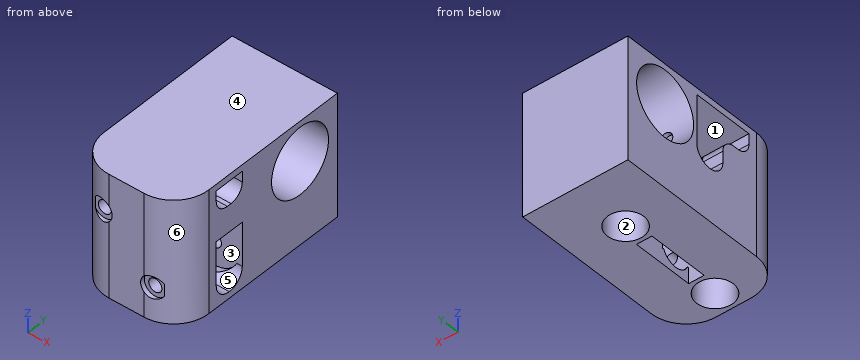
```python
from build123d import *

# Parameters (mm, degrees)
SKETCH_1_W           = 24
SKETCH_1_H           = 36
EXTRUDE_1_DEPTH      = 19
CUT_EXTRUDE_2_DEPTH  = 3.5
SKETCH_4_W           = 5.4
SKETCH_4_H           = 7
CUT_EXTRUDE_3_DEPTH  = 36.510561809
CUT_EXTRUDE_4_DEPTH  = 3.5
SKETCH_6_R           = 4.15
CUT_EXTRUDE_5_DEPTH  = 44.726422218
FILLET_2_R           = 3
SKETCH_10_W          = 10
SKETCH_10_H          = 36
CUT_EXTRUDE_9_DEPTH  = 36.510561809
SKETCH_11_W          = 28
SKETCH_11_H          = 16.5
EXTRUDE_3_DEPTH      = 24
SKETCH_12_W          = 10.25
SKETCH_12_H          = 12
EXTRUDE_4_DEPTH      = 7
FILLET_3_R           = 3.5
SKETCH_13_W          = 10.25
SKETCH_13_H          = 1.5
EXTRUDE_5_DEPTH      = 7
FILLET_4_R           = 3.5
SKETCH_14_R          = 5.6
CUT_EXTRUDE_10_DEPTH = 7
FILLET_6_R           = 3
EXTRUDE_START        = -18
SKETCH_16_R          = 4.15
EXTRUDE_6_DEPTH      = 18
SKETCH_17_R          = 7.65
SKETCH_17_W          = 28
SKETCH_17_H          = 17.5
SKETCH_17_H_2        = 9
CUT_EXTRUDE_11_DEPTH = 47.122120558
FILLET_7_R           = 8
SKETCH_18_R          = 1.5
CUT_EXTRUDE_12_DEPTH = 26
SKETCH_19_R          = 1.5
CUT_EXTRUDE_13_DEPTH = 20
SKETCH_20_R          = 2.5
CUT_EXTRUDE_14_DEPTH = 1


with BuildPart() as part:
    # 草图1 → 凸台-拉伸1 (new, symmetric)
    with BuildSketch(Plane.XY):
        Rectangle(SKETCH_1_W, SKETCH_1_H)
    extrude(amount=EXTRUDE_1_DEPTH, both=True)

    # 草图3 → 切除-拉伸2 (cut, symmetric)
    with BuildSketch(Plane(origin=(0, 3.5, 0), x_dir=(1, 0, 0), z_dir=(0, 1, 0))):
        with BuildLine():
            Line((-5.75, -7.5), (-12, -7.5))
            Line((-12, -7.5), (-12, 19))
            Line((-12, 19), (1.75, 19))
            Line((1.75, 19), (1.75, 0))
            ThreePointArc((1.75, 0), (-0.446699141, -5.303300859), (-5.75, -7.5))
        make_face()
    extrude(amount=CUT_EXTRUDE_2_DEPTH, both=True, mode=Mode.SUBTRACT)

    # 草图4 → 切除-拉伸3 (cut, through all)
    with BuildSketch(Plane.ZY.offset(12)):
        with Locations((4.8, -3.5)):
            Rectangle(SKETCH_4_W, SKETCH_4_H)
    extrude(amount=-CUT_EXTRUDE_3_DEPTH, mode=Mode.SUBTRACT)

    # 草图5 → 切除-拉伸4 (cut, symmetric)
    with BuildSketch(Plane(origin=(0, -3.5, 0), x_dir=(1, 0, 0), z_dir=(0, 1, 0))):
        with BuildLine():
            Line((5.75, 4), (12, 4))
            Line((12, 4), (12, 19))
            Line((12, 19), (-1.75, 19))
            Line((-1.75, 19), (-1.75, 11.5))
            ThreePointArc((-1.75, 11.5), (0.446699141, 6.196699141), (5.75, 4))
        make_face()
    extrude(amount=CUT_EXTRUDE_4_DEPTH, both=True, mode=Mode.SUBTRACT)

    # 草图6 → 切除-拉伸5 (cut, through all)
    with BuildSketch(Plane(origin=(0, 0, -19), x_dir=(-1, 0, 0), z_dir=(0, 0, -1))):
        with Locations((0, 12)):
            Circle(SKETCH_6_R)
        with Locations(Location((0, -12, 0), (0, 0, 180))):
            Circle(SKETCH_6_R)
    extrude(amount=-CUT_EXTRUDE_5_DEPTH, mode=Mode.SUBTRACT)

    # 圆角2
    fillet_2_edges = [part.edges().sort_by_distance(p)[0] for p in [
        (6.725, 0, 2.1),
        (0, -7, 2.1),
    ]]
    fillet(fillet_2_edges, radius=FILLET_2_R)

    # 草图10 → 切除-拉伸9 (cut, through all)
    with BuildSketch(Plane(origin=(12, 0, 0), x_dir=(0, 0, -1), z_dir=(1, 0, 0))):
        with Locations((-14, 0)):
            Rectangle(SKETCH_10_W, SKETCH_10_H)
    extrude(amount=-CUT_EXTRUDE_9_DEPTH, mode=Mode.SUBTRACT)

    # 草图11 → 凸台-拉伸3 (add)
    with BuildSketch(Plane.ZY.offset(12)):
        with Locations((-5, -26.25)):
            Rectangle(SKETCH_11_W, SKETCH_11_H)
    extrude_3 = extrude(amount=-EXTRUDE_3_DEPTH)

    # 镜向2: 凸台-拉伸3 across plane
    add(extrude_3.mirror(Plane.ZX))

    # 草图12 → 凸台-拉伸4 (add)
    with BuildSketch(Plane(origin=(0, 0, 0), x_dir=(1, 0, 0), z_dir=(0, 1, 0))):
        with Locations((-6.875, 13)):
            Rectangle(SKETCH_12_W, SKETCH_12_H)
    extrude(amount=EXTRUDE_4_DEPTH)

    # 圆角3
    fillet_3_edges = [part.edges().sort_by_distance(p)[0] for p in [
        (-6.875, 0, -7),
        (-6.875, 7, -7),
    ]]
    fillet(fillet_3_edges, radius=FILLET_3_R - 0.0001)  # a hair under: the kernel refuses the full size

    # 草图13 → 凸台-拉伸5 (add)
    with BuildSketch(Plane.XZ):
        with Locations((6.875, -18.25)):
            Rectangle(SKETCH_13_W, SKETCH_13_H)
    extrude(amount=EXTRUDE_5_DEPTH)

    # 圆角4
    fillet_4_edges = [part.edges().sort_by_distance(p)[0] for p in [
        (6.875, 0, -17.5),
        (6.875, -7, -17.5),
    ]]
    fillet(fillet_4_edges, radius=FILLET_4_R - 0.0001)  # a hair under: the kernel refuses the full size

    # 草图14 → 切除-拉伸10 (cut)
    with BuildSketch(Plane.XZ):
        with Locations((5.75, -11.5)):
            Circle(SKETCH_14_R)
    extrude(amount=CUT_EXTRUDE_10_DEPTH, mode=Mode.SUBTRACT)

    # 圆角6
    fillet_6_edges = [part.edges().sort_by_distance(p)[0] for p in [
        (-5.275, 0, 2.1),
    ]]
    fillet(fillet_6_edges, radius=FILLET_6_R)

    # 草图16 → 凸台-拉伸6 (add)
    with BuildSketch(Plane.XY.offset(9).offset(EXTRUDE_START)):
        with Locations((0, -12)):
            Circle(SKETCH_16_R)
        with Locations(Location((0, 12, 0), (0, 0, 180))):
            Circle(SKETCH_16_R)
    extrude(amount=EXTRUDE_6_DEPTH)

    # 草图17 → 切除-拉伸11 (cut, through all)
    with BuildSketch(Plane.ZY.offset(12)):
        with Locations(Location((0, 15.5, 0), (0, 0, 270))):
            Circle(SKETCH_17_R)
        with Locations((-5, -25.75)):
            Rectangle(SKETCH_17_W, SKETCH_17_H)
        with Locations((-5, 30)):
            Rectangle(SKETCH_17_W, SKETCH_17_H_2)
    extrude(amount=-CUT_EXTRUDE_11_DEPTH, mode=Mode.SUBTRACT)

    # 圆角7
    fillet_7_edges = [part.edges().sort_by_distance(p)[0] for p in [
        (12, -17, -5),
        (-12, -17, -5),
    ]]
    fillet(fillet_7_edges, radius=FILLET_7_R)

    # 草图18 → 切除-拉伸12 (cut)
    with BuildSketch(Plane.XZ.offset(17)):
        with Locations((-5.75, 0)):
            Circle(SKETCH_18_R)
    extrude(amount=-CUT_EXTRUDE_12_DEPTH, mode=Mode.SUBTRACT)

    # 草图19 → 切除-拉伸13 (cut)
    with BuildSketch(Plane.XZ.offset(17)):
        with Locations((5.75, -11.5)):
            Circle(SKETCH_19_R)
    extrude(amount=-CUT_EXTRUDE_13_DEPTH, mode=Mode.SUBTRACT)

    # 草图20 → 切除-拉伸14 (cut)
    with BuildSketch(Plane.XZ.offset(17)):
        with Locations((5.75, -11.5)):
            Circle(SKETCH_20_R)
        with Locations((-5.75, 0)):
            Circle(SKETCH_20_R)
    extrude(amount=-CUT_EXTRUDE_14_DEPTH, mode=Mode.SUBTRACT)


solid = part.part
```
Could you check a few things on this model? Use its own coordinates, in mm. Face numbers are marked on the shaded views. A direction names the side the tool comes from. Give positions to 0.01 mm unless a question says otherwise; leave off trailing zeros. Order: outer loops, then holes, each group sorted by start corner. A loop starts at its lowest first (then second) coordinate and runs counter-clockwise, first axis right, second up.
Q1. For the marked faces 1, 2 and 3, which set-ups out of +Z, -Z, +X, -X, +Y, -Y let a thin tool reach every point of the face, with its end or its side?
Q2. Suppose I cut it at D-D, the plane z = -8.5. Write out the boundary of the cut face in (x, y).
Q3. If I drill on line 1 along Y through (x, z) = (0, -11.75); line 2 along X through (y, z) = (12, -12.25); line 3 along Y through (x, z) = (2, -0.25), over which ranges is the centre line in solid material (lowest first)?
Q4. I'm going to push a flat-ended pin straight in: P1, Ø2.5, axis at x = 6.5, z = -11, coming from the -Y side. Where does the tip first touch, or does it pass through?
Q5. Suppose I cut it at B-B, the plane y = -6. Write out the boundary of the cut face in (x, z), and give its area (3 significant figures).
Q6. We'd pull the mould along Y, two halves only. Please class the marked faces 4, 5 and 6: +Y half, -Y half, draft (parallel to the pull), parting line (faces both ways), or undercut.
Q7. Suppose I cut it at C-C, the plane z = 4.25. Write out the boundary of the cut face in (x, y), and give its area (3 significant figures).
Q8. Suppose I cut it at A-A, the plane y = 5.5. Write out the boundary of the cut face in (x, z), and give its area (3 significant figures).
Solution:
1. face 1: -X
1. face 2: -Z
1. face 3: none
2. outline: (-12, -9) arc R8 ccw to (-4, -17) - (4, -17) arc R8 ccw to (12, -9) - (12, -7) - (-1.12, -7) - (-1.12, 0) - (-1.75, 0) - (-1.75, 7) - (1.75, 7) - (1.75, 0) - (12, 0) - (12, 25.5) - (-12, 25.5) - close
3. line 1: y = -17 to -16.15, -7.85 to -7, 7 to 7.85, 16.15 to 25.5
3. line 2: x = -12 to -4.15, 4.15 to 12
3. line 3: y = -17 to 7.85, 23.15 to 25.5
4. P1: stops at y = -16
5. outline: (-12, -19) - (-1.75, -19) - (-1.75, -11.5) arc R7.5 cw to (5.75, -4) - (12, -4) - (12, 2.86) - (-12, 2.86) - close; (-12, 7.5) - (12, 7.5) - (12, 9) - (-12, 9) - close; (1.75, -19) - (12, -19) - (12, -16.45) - (8.37, -16.45) arc R5.6 cw to (3.13, -16.45) - (1.75, -16.45) - close; hole circle Ø3 at (-5.75, 0)
5. area: 383 mm2
6. face 4: draft
6. face 5: undercut
6. face 6: -Y half
7. outline: (-12, -9) arc R8 ccw to (-4, -17) - (4, -17) arc R8 ccw to (12, -9) - (12, -6.88) - (-12, -6.88) - close; (-12, 7) - (0.43, 7) - (0.43, -0.12) - (12, -0.12) - (12, 9.14) - (-12, 9.14) - close; (-12, 21.86) - (12, 21.86) - (12, 25.5) - (-12, 25.5) - close
7. area: 437 mm2
8. outline: (-12, -19) - (-1.75, -19) - (-1.75, -6.37) - (-12, -6.37) - close; (-12, 7.5) - (-5.75, 7.5) arc R7.5 cw to (1.75, 0) - (1.75, -19) - (12, -19) - (12, 9) - (-12, 9) - close
8. area: 449 mm2
